Geometry check sheet. Reference: the model listing, model coordinates, mm. Face numbers are marked on the shaded views. A direction names the side the tool comes from. Give positions to 0.01 mm unless a question says otherwise; leave off trailing zeros. Write each loop counter-clockwise with the first axis right and the second up, starting at its lowest first coordinate (ties: lowest second). Pieces come first, ordered by that corner, then holes. Notation, with made-up numbers: (29, -16) -> (74, -16) arc R19 ccw to (74, 19) -> close; hole circle Ø3 at (71.25, 69). An arc over 180 degrees is marked (long way). One line per item, written item: value.
from build123d import *

# Parameters (mm, degrees)
CHAMFER1_SIZE            = 4
FILLET1_R                = 3.5
BOSS_EXTRUDE1_DEPTH      = 90
BOSS_EXTRUDE1_DEPTH_BACK = 80
SKETCH2_R                = 37.5
BOSS_EXTRUDE2_START      = 60
BOSS_EXTRUDE2_DEPTH      = 12.5
SKETCH4_R                = 9.5
BOSS_EXTRUDE3_DEPTH      = 9.5
SKETCH5_R                = 55
BOSS_EXTRUDE4_DEPTH      = 30
SKETCH6_R                = 7.5
BOSS_EXTRUDE5_DEPTH      = 25
BOSS_EXTRUDE6_START      = 6
SKETCH6_3_R              = 7.5
BOSS_EXTRUDE6_DEPTH      = 12.5
CIRPATTERN2_COUNT        = 15


with BuildPart() as part:
    # Sketch1 → Revolve1 (revolve)
    with BuildSketch(Plane(origin=(0, 0, 0), x_dir=(0, 0, -1), z_dir=(1, 0, 0))):
        Polygon((0, 0), (0, 165), (95, 165), (133, 154.817930688), (133, 75), (158, 75), (158, 50), (183, 50), (183, 0), align=None)
    revolve(axis=Axis((0, 0, -183), (0, 0, 1)))

    # Chamfer1
    chamfer1_edges = [part.edges().sort_by_distance(p)[0] for p in [
        (0, -50, -183),
    ]]
    chamfer(chamfer1_edges, length=CHAMFER1_SIZE)

    # Fillet1
    fillet1_edges = [part.edges().sort_by_distance(p)[0] for p in [
        (0, -50, -158),
        (0, -75, -158),
    ]]
    fillet(fillet1_edges, radius=FILLET1_R)



with BuildPart() as body_2:
    # Sketch2 → Boss-Extrude1 (new, two sides: drawn at the far end of the back side and taken through both)
    with BuildSketch(Plane(origin=(0, 0, 0), x_dir=(1, 0, 0), z_dir=(0, 1, 0)).offset(-BOSS_EXTRUDE1_DEPTH_BACK)):
        with Locations(Location((0, -75, 0), (0, 0, 270))):
            Circle(SKETCH2_R)
    extrude(amount=BOSS_EXTRUDE1_DEPTH + BOSS_EXTRUDE1_DEPTH_BACK)


with BuildPart() as part_1:
    add(part.part)

    add(body_2.part)  # Boss-Extrude2 merges body 2
    # Sketch3 → Boss-Extrude2 (add)
    with BuildSketch(Plane(origin=(0, 0, 0), x_dir=(1, 0, 0), z_dir=(0, 1, 0)).offset(BOSS_EXTRUDE2_START)):
        Polygon((-50, 0), (50, 0), (50, -25), (36.542960266, -83.417960266), (-36.542960266, -83.417960266), (-50, -25), align=None)
    boss_extrude2 = extrude(amount=-BOSS_EXTRUDE2_DEPTH)

    # Mirror1: Boss-Extrude2 across plane
    add(boss_extrude2.mirror(Plane.ZX))

    # Sketch4 → Boss-Extrude3 (add, symmetric)
    with BuildSketch(Plane(origin=(0, 0, 0), x_dir=(1, 0, 0), z_dir=(0, 1, 0))):
        with BuildLine():
            Line((-50, 0), (100, 0))
            Line((100, 0), (100, -25))
            Line((100, -25), (37.5, -75))
            ThreePointArc((37.5, -75), (0, -112.5), (-37.5, -75))
            Line((-37.5, -75), (-150, -75))
            ThreePointArc((-150, -75), (-174.822997079, -52.969649142), (-155.897247359, -25.705505282))
            Line((-155.897247359, -25.705505282), (-50, 0))
        make_face()
        with Locations(Location((-150, -50, 0), (0, 0, 270))):
            Circle(SKETCH4_R, mode=Mode.SUBTRACT)
    extrude(amount=BOSS_EXTRUDE3_DEPTH, both=True)

    # Sketch5 → Boss-Extrude4 (add)
    with BuildSketch(Plane(origin=(0, 60, 0), x_dir=(1, 0, 0), z_dir=(0, 1, 0))):
        with Locations(Location((0, -75, 0), (0, 0, 145.958125966))):
            Circle(SKETCH5_R)
    extrude(amount=BOSS_EXTRUDE4_DEPTH)

    # Sketch6 → Boss-Extrude5 (add)
    with BuildSketch(Plane(origin=(0, 0, -133), x_dir=(-1, 0, 0), z_dir=(0, 0, -1))):
        with Locations(Location((0, 120, 0), (0, 0, 90))):
            Circle(SKETCH6_R)
    boss_extrude5 = extrude(amount=BOSS_EXTRUDE5_DEPTH)

    # Sketch6<3> → Boss-Extrude6 (add)
    with BuildSketch(Plane(origin=(0, 0, -133), x_dir=(-1, 0, 0), z_dir=(0, 0, -1)).offset(BOSS_EXTRUDE6_START)):
        Polygon((7.216878365, 132.5), (-7.216878365, 132.5), (-14.43375673, 120), (-7.216878365, 107.5), (7.216878365, 107.5), (14.43375673, 120), align=None)
        with Locations((0, 120)):
            Circle(SKETCH6_3_R, mode=Mode.SUBTRACT)
    boss_extrude6 = extrude(amount=BOSS_EXTRUDE6_DEPTH)

    # CirPattern2: Boss-Extrude5, Boss-Extrude6 ×15 about axis
    cirpattern2_axis = Axis((0, 0, 0), (0, 0, 1))
    add([boss_extrude5.rotate(cirpattern2_axis, i * 360 / CIRPATTERN2_COUNT) for i in range(1, CIRPATTERN2_COUNT)])
    add([boss_extrude6.rotate(cirpattern2_axis, i * 360 / CIRPATTERN2_COUNT) for i in range(1, CIRPATTERN2_COUNT)])


solid = part_1.part
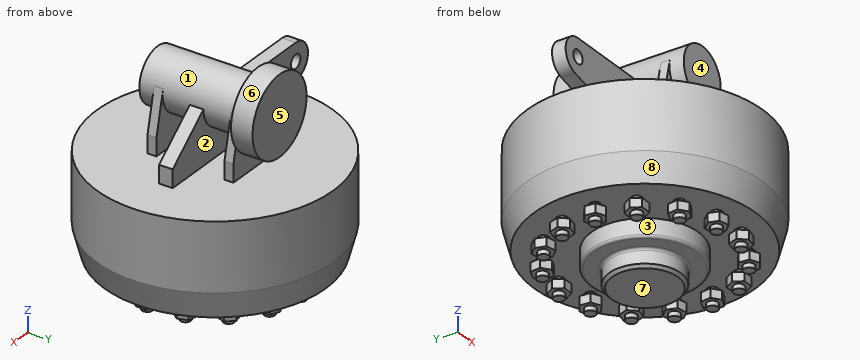
1) Tool access check on the marked faces 4, 5, 6, 7 and 8. Record the directions out of +Z, -Z, +X, -X, +Y, -Y that give a thin tool (end or side, any length) a straight path to the whole face; none if there is none.
Verdict:
face 4: +Z, +X, -X, -Y
face 5: +Z, +X, -X, +Y
face 6: +Y
face 7: -Z, +X, -X, +Y, -Y
face 8: -Z
2) Sectioned sample at A-A on x = 0. Give the number of separate pieces and of enclosed holes in the cut face, plus the area to 3 significant figures.
Verdict:
separate pieces: 1
enclosed holes: 2
area: 65,700 mm^2
3) Scan lines: probe 1 along Y at (x, z) = (-27, 42.5); probe 2 along Z at (x, y) = (-151, -6.5); probe 3 along Z at (x, y) = (-151, 15). Record each from-to range of solid material in increasing order.
Verdict:
probe 1: -60 to -47.5, -9.5 to 9.5, 47.5 to 90
probe 2: -133 to 0, 24.52 to 40.55, 59.45 to 74.98
probe 3: -133 to 0
4) Depth check by flat-ended pin: pin 1 Ø21 at (x, y) = (-49.5, 114) entering from +Z; pin 2 Ø1.5 at (y, z) = (38, -146) entering from -X; pin 3 Ø8 at (x, y) = (88.5, 78) entering from -Z. Enter the tip coordinate at first touch or a pass-through.
Verdict:
pin 1: z = 0
pin 2: x = -127.22
pin 3: z = -158
5) Sectioned sample at D-D on z = 107.5. Record the cut outline in (x, y).
Verdict:
outline: (-44.37, 60) -> (-18.71, 60) -> (-18.71, -80) -> (18.71, -80) -> (18.71, 60) -> (44.37, 60) -> (44.37, 90) -> (-44.37, 90) -> close
6) Sectioned sample at C-C on z = -84.5. Record the cut outline in (x, y).
Verdict:
outline: circle Ø330 at (0, 0)
7) Mould release check, pull along X, two halves, no side actions. Record for the marked faces 1, 2 and 3: released by +X, released by -X, zero draft, split by the parting line, or undercut.
Verdict:
face 1: split by the parting line
face 2: zero draft
face 3: undercut
